from build123d import *

# Parameters (mm, degrees)
EXTRUDE_THIN1_DEPTH                                 = 25.4
CUT_EXTRUDE1_DEPTH                                  = 111.716033166
CBORE_FOR_00_BINDING_HEAD_MACHINE_SCREW_D           = 6.35
CBORE_FOR_00_BINDING_HEAD_MACHINE_SCREW_CBORE_D     = 12.7
CBORE_FOR_00_BINDING_HEAD_MACHINE_SCREW_CBORE_DEPTH = 3.302
RIB1_REACH                                          = 112.716
SKETCH6_WALL_W                                      = 287.08428389
SKETCH6_WALL_H                                      = 6.35
FILLET1_R                                           = 12.7
FILLET2_R                                           = 1.524
FILLET3_RADIUS                                      = 25.4
FILLET3_LENGTH                                      = 9.652
FILLET4_R                                           = 1.524


with BuildPart() as part:
    # Sketch2 → Extrude-Thin1 (new, symmetric)
    with BuildSketch(Plane.XY):
        Polygon((-35.921024484, 35.921024484), (0, 0), (101.6, 0), (101.6, -9.652), (-3.997989304, -9.652), (-42.746019136, 29.096029832), align=None)
    extrude(amount=EXTRUDE_THIN1_DEPTH, both=True)

    # Sketch3 → Cut-Extrude1 (cut, through all)
    with BuildSketch(Plane(origin=(0, 0, 0), x_dir=(1, 0, 0), z_dir=(0, 1, 0))):
        with BuildLine():
            Line((50.8, 12.7), (76.2, 12.7))
            ThreePointArc((76.2, 12.7), (88.9, 0), (76.2, -12.7))
            Line((76.2, -12.7), (50.8, -12.7))
            ThreePointArc((50.8, -12.7), (38.1, 0), (50.8, 12.7))
        make_face()
    extrude(amount=-CUT_EXTRUDE1_DEPTH, mode=Mode.SUBTRACT)

    # CBORE for #00 Binding Head Machine Screw1 (through all)
    with Locations(Plane(origin=(0, 0, 0), x_dir=(0.7071067811865513, -0.7071067811865438, 0), z_dir=(0.7071067811865438, 0.7071067811865513, 0))):
        with Locations((-38.1, -12.7)):
            cbore_for_00_binding_head_machine_screw = CounterBoreHole(CBORE_FOR_00_BINDING_HEAD_MACHINE_SCREW_D / 2, CBORE_FOR_00_BINDING_HEAD_MACHINE_SCREW_CBORE_D / 2, CBORE_FOR_00_BINDING_HEAD_MACHINE_SCREW_CBORE_DEPTH)

    # Mirror1: CBORE for #00 Binding Head Machine Screw1 across plane
    add(cbore_for_00_binding_head_machine_screw.mirror(Plane.XY), mode=Mode.SUBTRACT)

    # Sketch6 wall → Rib1 (add, up to next)
    with BuildSketch(Plane(origin=(-2.54, 15.24, 0), x_dir=(0.877895572914, -0.478852130681, 0), z_dir=(0.478852130681, 0.877895572914, 0)), mode=Mode.PRIVATE) as rib1_sk1:
        Rectangle(SKETCH6_WALL_W, SKETCH6_WALL_H)
    rib1_tool1 = extrude(rib1_sk1.sketch, amount=-RIB1_REACH, mode=Mode.PRIVATE) - part.part
    add(rib1_tool1.solids().sort_by_distance((-2.54, 15.24, 0))[0])

    # Fillet1
    fillet1_edges = [part.edges().sort_by_distance(p)[0] for p in [
        (-39.33352181, 32.508527158, -25.4),
        (-39.33352181, 32.508527158, 25.4),
    ]]
    fillet(fillet1_edges, radius=FILLET1_R)

    # Fillet2
    fillet2_edges = [part.edges().sort_by_distance(p)[0] for p in [
        (0, 0, -14.2875),
        (0, 0, 14.2875),
        (-3.997989304, -9.652, 0),
    ]]
    fillet(fillet2_edges, radius=FILLET2_R)

    # Fillet3: full round fillet: the end face becomes a half cylinder, R = half its width
    fillet3_face = Plane((101.6, -4.826, 0), x_dir=(0, -1, 0), z_dir=(1, 0, 0))  # on the end face: x along it, z out of the body
    fillet3_slab = fillet3_face.offset(-FILLET3_RADIUS / 2) * Box(FILLET3_LENGTH, 2 * FILLET3_RADIUS, FILLET3_RADIUS, mode=Mode.PRIVATE)  # the body's end, R deep
    fillet3_round = Plane((76.2, -4.826, 0), x_dir=(1, 0, 0), z_dir=(0, -1, 0)) * Cylinder(FILLET3_RADIUS, FILLET3_LENGTH, mode=Mode.PRIVATE)  # its axis R under the face
    add(fillet3_slab - fillet3_round, mode=Mode.SUBTRACT)

    # Fillet4
    fillet4_edges = [part.edges().sort_by_distance(p)[0] for p in [
        (38.415630735, 0, 25.4),
        (38.415630735, 0, -25.4),
        (101.6, 0, 0),
        (-35.921024484, 35.921024484, 0),
        (-33.290768363, 33.290768363, 21.680256121),
        (-33.290768363, 33.290768363, -21.680256121),
        (-13.693568814, 13.693568814, -25.4),
        (-13.693568814, 13.693568814, 25.4),
        (0.048051918, 0.116007592, -25.4),
        (0.048051918, 0.116007592, 25.4),
    ]]
    fillet(fillet4_edges, radius=FILLET4_R)


solid = part.part
CAD build for the part. Positions are in the model's coordinates, mm. A direction names the side the tool comes from. Round coordinates to 2 decimals unless told otherwise and drop trailing zeros. Write each loop counter-clockwise with the first axis right and the second up, starting at its lowest first coordinate (ties: lowest second). Pieces come first, ordered by that corner, then holes. Notation, with made-up numbers: (63.25, 10) -> (95.25, 10) arc R15 ccw to (95.25, 39) -> close; hole circle Ø3 at (30, 63). An arc over 180 degrees is marked (long way). Answer as a JSON object with one key per item and string values.
(1) Band-saw the part on A-A, the plane x = 66.5. List the corners of the cut face in (y, z), then the cut area to 3 significant figures.
Reported:
{"outline": "(-9.65, -25.4) -> (-1.52, -25.4) arc R1.52 ccw to (0, -23.88) -> (0, -12.7) -> (-9.65, -12.7) -> close; (-9.65, 12.7) -> (0, 12.7) -> (0, 23.88) arc R1.52 ccw to (-1.52, 25.4) -> (-9.65, 25.4) -> close", "area": "244 mm^2"}
(2) Band-saw the part on C-C, the plane x = 4. List the corners of the cut face in (y, z) (3 decimals), then the cut area to 3 significant figures.
Reported:
{"outline": "(-9.652, -25.4) -> (-1.524, -25.4) arc R1.524 ccw to (0, -23.876) -> (0, -3.175) -> (11.673, -3.175) -> (11.673, 3.175) -> (0, 3.175) -> (0, 23.876) arc R1.524 ccw to (-1.524, 25.4) -> (-9.652, 25.4) -> close", "area": "563 mm^2"}
(3) Which spindle directions (+Z, -Z, +X, -X, +Y, -Y) get a long thin tool onto all of the face, cutting with end or side? Do faces 4 (the face through (38.6, 0, -5)), 5 (the face through (-27.34, 22.67, 15.43)), 6 (the face through (63, -5, -12.7)). Say none if no direction does.
Reported:
{"face 4": "+X, +Y", "face 5": "none", "face 6": "+Y, -Y"}
(4) Probe probe 1 along Y at (x, z) = (7, -4); probe 2 along X at (y, z) = (-4, -7); probe 3 along X at (y, z) = (19, 12.5). List the from-to ranges inside material, lowest first. Write a range as [from, to].
Reported:
{"probe 1": "y = [-9.65, 0]", "probe 2": "x = [-9.65, 40.2], [86.8, 100.62]", "probe 3": "x = [-30.4, -19]"}
(5) Pin check, flat tips, straight feed: P1, Ø6, axis at x = 48, y = 2.5, coming from the +Z side; P2, Ø6, axis at y = 24, z = 7, coming from the -X side; P3, Ø14.5, axis at x = 29, z = -11, coming from the +Y side. Stop position of each tip, or through.
Reported:
{"P1": "stops at z = 25", "P2": "stops at x = -40.65", "P3": "stops at y = 0"}
(6) Band-saw the part on B-B, the plane z = 0. List the corners of the cut face in (x, y), then the cut area to 3 significant figures.
Reported:
{"outline": "(-42.75, 29.1) -> (-4.44, -9.21) arc R1.52 ccw to (-3.37, -9.65) -> (38.1, -9.65) -> (38.1, 0) -> (25.4, 0) -> (-30.48, 30.48) -> (-34.84, 34.84) arc R1.52 ccw to (-37, 34.84) -> close; (88.9, -9.65) -> (101.6, -9.65) -> (101.6, -1.52) arc R1.52 ccw to (100.08, 0) -> (88.9, 0) -> close", "area": "1,410 mm^2"}
(7) Two-plate mould, pull along Z, no slides. Class faces 1 (the face through (-37.27, 29.45, 21.58)), 2 (the face through (-27.34, 22.67, -15.43)), 3 (the face through (-23.33, 9.68, 0.36)): +Z half, -Z half, draft (parallel to the pull), parting line (faces both ways), or undercut.
Reported:
{"face 1": "+Z half", "face 2": "undercut", "face 3": "draft"}
